Verification items for this drawing (mm, ordinates from the low corner). Round coordinates to 2 decimals unless told otherwise and drop trailing zeros. Loops run counter-clockwise (first coordinate to the right, second up) from the corner with the lowest first, then second, coordinate; pieces in that order, holes last. Notation, with made-up numbers: (-23.75, -8) - (14.25, -8) arc R11 cw to (14.25, 4) - close; hole circle Ø3 at (-22.75, -23). An arc over 180 degrees is marked (long way). Answer in a Markdown table with one row per item. Add a question column.
(1) Cross-section at C-C on y = 5.75. Enter the section's corners in (x, z).
(2) Thickness scan on line 1 along X through (y, z) = (1.75, 27); line 2 along X through (y, z) = (6.5, 5); line 3 along Z through (x, y) = (136, 4.25). Record the ranges inside material, lowest first.
(3) Gauge pin test, flat end, axial feed: pin 1 (6.5 mm diameter, centred on x = 95, z = 75, fed in from -Y). Record the tip position at first contact, or that the pin passes through.
(4) Cross-section at A-A on z = 5. Enter the section's corners in (x, y).
(5) Cross-section at B-B on x = 51.5. Enter the section's corners in (y, z), then the cut area to 3 significant figures.
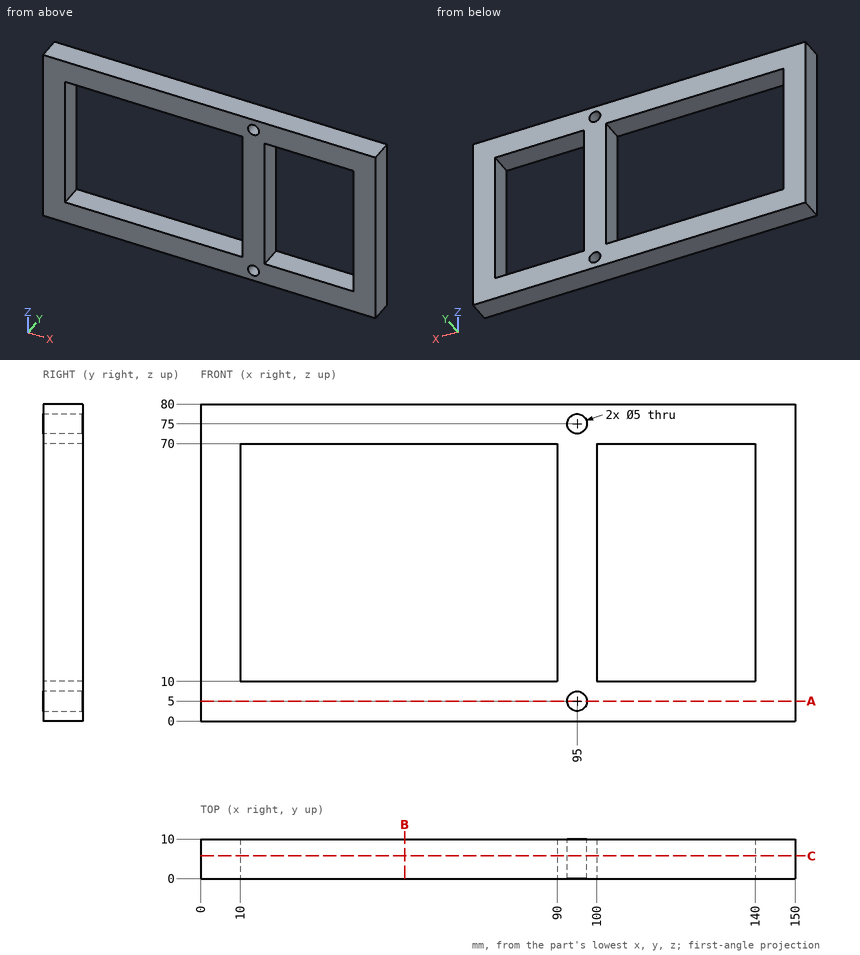
Answers:
| question | item | result |
|---|---|---|
| 1 | outline | (0, 0) - (150, 0) - (150, 80) - (0, 80) - close; hole (10, 10) - (90, 10) - (90, 70) - (10, 70) - close; hole circle Ø5 at (95, 5); hole circle Ø5 at (95, 75); hole (100, 10) - (140, 10) - (140, 70) - (100, 70) - close |
| 2 | line 1 | x = 0 to 10, 90 to 100, 140 to 150 |
| 2 | line 2 | x = 0 to 92.5, 97.5 to 150 |
| 2 | line 3 | z = 0 to 10, 70 to 80 |
| 3 | pin 1 | stops at y = 0 |
| 4 | outline | (0, 0) - (92.5, 0) - (92.5, 10) - (0, 10) - close; (97.5, 0) - (150, 0) - (150, 10) - (97.5, 10) - close |
| 5 | outline | (0, 0) - (10, 0) - (10, 10) - (0, 10) - close; (0, 70) - (10, 70) - (10, 80) - (0, 80) - close |
| 5 | area | 200 mm^2 |
